```python
from build123d import *

# Parameters (mm, degrees)
SKETCH1_W           = 40
SKETCH1_H           = 40
BOSS_EXTRUDE1_DEPTH = 23.5
CHAMFER1_SIZE       = 2
SKETCH2_R           = 11
BOSS_EXTRUDE2_DEPTH = 1
SKETCH3_R           = 2.5
BOSS_EXTRUDE3_DEPTH = 15


with BuildPart() as part:
    # Sketch1 → Boss-Extrude1 (new body, symmetric)
    with BuildSketch(Plane.XY):
        Rectangle(SKETCH1_W, SKETCH1_H)
    extrude(amount=BOSS_EXTRUDE1_DEPTH, both=True)

    # Chamfer1
    chamfer1_edges = [part.edges().sort_by_distance(p)[0] for p in [
        (-20, 0, 23.5),
        (0, -20, 23.5),
        (20, 0, 23.5),
        (0, -20, -23.5),
        (-20, 0, -23.5),
        (0, 20, -23.5),
        (20, 0, -23.5),
        (20, -20, 0),
        (-20, -20, 0),
        (-20, 20, 0),
        (20, 20, 0),
        (0, 20, 23.5),
    ]]
    chamfer(chamfer1_edges, length=CHAMFER1_SIZE)

    # Sketch2 → Boss-Extrude2 (add, symmetric)
    with BuildSketch(Plane(origin=(0, 0, -23.5), x_dir=(-1, 0, 0), z_dir=(0, 0, -1))):
        Circle(SKETCH2_R)
    extrude(amount=BOSS_EXTRUDE2_DEPTH, both=True)

    # Sketch3 → Boss-Extrude3 (add, symmetric)
    with BuildSketch(Plane(origin=(0, 0, -24.5), x_dir=(-1, 0, 0), z_dir=(0, 0, -1))):
        Circle(SKETCH3_R)
    extrude(amount=BOSS_EXTRUDE3_DEPTH, both=True)


solid = part.part
```
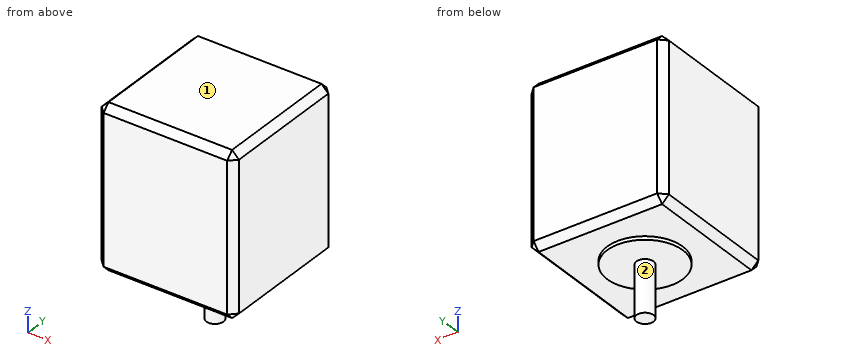
Geometry check sheet. Reference: the model listing, model coordinates, mm. Face numbers are marked on the shaded views. A direction names the side the tool comes from. Give positions to 0.01 mm unless a question says otherwise; leave off trailing zeros. Loops run counter-clockwise (first coordinate to the right, second up) from the corner with the lowest first, then second, coordinate; pieces in that order, holes last. Notation, with made-up numbers: M 11,23 L 19,23 A8 ccw 19,30 Z; hole C 48.5,-21.75 d8. An arc over 180 degrees is marked long. Answer as CSV lines item,"result".
Item 1: Material ranges on line 1 (Z direction, x = 16, y = 1.5); line 2 (Z direction, x = 3.5, y = 9.5); line 3 (X direction, y = -0.5, z = -33), recorded low to high.
Values:
line 1,"z = -23.5 to 23.5"
line 2,"z = -24.5 to 23.5"
line 3,"x = -2.45 to 2.45"
Item 2: Access from +Z, -Z, +X, -X, +Y, -Y to the whole of each face (thin tool, end or side, straight path). Record for the marked faces 1 and 2.
Values:
face 1,"+Z, +X, -X, +Y, -Y"
face 2,"-Z"
Item 3: Cross-section at C-C on x = 17. Record the cut outline in (y, z).
Values:
outline,"M -20,-21.5 L -18,-23.5 L 18,-23.5 L 20,-21.5 L 20,21.5 L 18,23.5 L -18,23.5 L -20,21.5 Z"
Item 4: Cross-section at A-A on y = 0. Record the cut outline in (x, z).
Values:
outline,"M -20,-21.5 L -18,-23.5 L -11,-23.5 L -11,-24.5 L -2.5,-24.5 L -2.5,-39.5 L 2.5,-39.5 L 2.5,-24.5 L 11,-24.5 L 11,-23.5 L 18,-23.5 L 20,-21.5 L 20,21.5 L 18,23.5 L -18,23.5 L -20,21.5 Z"
Item 5: Depth check by flat-ended pin: P1, Ø12, axis at y = -12.5, z = -32.5, coming from the -X side; P2, Ø1, axis at x = -6, y = -9, coming from the -Z side. Enter the tip coordinate at first touch or a pass-through.
Values:
P1,"passes through"
P2,"stops at z = -24.5"
